Read the model definition and answer for the solid it produces. Units are mm, in the model's axes. A direction names the side the tool comes from. Round coordinates to 2 decimals unless told otherwise and drop trailing zeros. Loops run counter-clockwise (first coordinate to the right, second up) from the corner with the lowest first, then second, coordinate; pieces in that order, holes last. Notation, with made-up numbers: (-16, -38.75) -> (41, -38.75) arc R19 ccw to (41, -31.75) -> close; hole circle Ø7 at (36, -27). An arc over 180 degrees is marked (long way). Put each result on its own line as item: value.
from build123d import *

# Parameters (mm, degrees)
F2_R     = 2.915028
F3_DEPTH = 25.4
F4_SIZE  = 0.8128
F5_R     = 1.809052
F6_DEPTH = 127.001


with BuildPart() as f1:
    # F0 (on Front) → F1 (revolve)
    with BuildSketch(Plane.XZ):
        Polygon((0, -50.8), (0, 0), (0, 76.2), (-6.35, 76.2), (-6.35, 0), (-25.4, 0), align=None)
    revolve(axis=Axis((0, 0, 38.1), (0, 0, -1)))

    # F2 (on face) → F3 (cut)
    with BuildSketch(Plane.XY.offset(76.2)):
        Circle(F2_R)
    extrude(amount=-F3_DEPTH, mode=Mode.SUBTRACT)

    # F4
    f4_edges = [f1.edges().sort_by_distance(p)[0] for p in [
        (6.35, 0, 76.2),
    ]]
    chamfer(f4_edges, length=F4_SIZE)

    # F5 (on face) → F6 (cut, through all)
    with BuildSketch(Plane.XY.offset(76.2)):
        Circle(F5_R)
    extrude(amount=-F6_DEPTH, mode=Mode.SUBTRACT)


solid = f1.part
Item 1: The part is cut by section D-D (z = 7.5). Determine the outline of the cut face in (x, y).
Derived:
outline: circle Ø12.7 at (0, 0); hole circle Ø3.62 at (0, 0)
Item 2: Flat-ended cylindrical pins translate along their axes: pin 1 Ø4 at (x, y) = (16.5, -13) entering from -Z; pin 2 Ø6 at (x, z) = (1.5, 0.5) entering from +Y; pin 3 Ø4 at (x, y) = (19, 14.5) entering from -Z. Find the tip coordinate at first contact, or state that the pin passes through.
Derived:
pin 1: stops at z = -12.79
pin 2: stops at y = 25.4
pin 3: stops at z = -7
Item 3: The part is cut by section A-A (x = 0). Determine the outline of the cut face in (y, z).
Derived:
outline: (-25.4, 0) -> (-1.81, -47.18) -> (-1.81, 50.8) -> (-2.92, 50.8) -> (-2.92, 76.2) -> (-5.54, 76.2) -> (-6.35, 75.39) -> (-6.35, 0) -> close; (1.81, -47.18) -> (25.4, 0) -> (6.35, 0) -> (6.35, 75.39) -> (5.54, 76.2) -> (2.92, 76.2) -> (2.92, 50.8) -> (1.81, 50.8) -> close
Item 4: The part is cut by section C-C (z = -30.5). Determine the outline of the cut face in (x, y).
Derived:
outline: circle Ø20.3 at (0, 0); hole circle Ø3.62 at (0, 0)
Item 5: For a pull along X with two mould halves and no side action, classify faces 1 (the flat face through (5, -5, 0)), 2 (the cylindrical face through (1.38, -6.2, 37.17)), 3 (the flat face through (0, -2, 50.8)) as pulls with the +X half, pulls with the -X half, needs draft (parallel to the pull), parting line crosses it, or undercut.
Derived:
face 1: needs draft
face 2: parting line crosses it
face 3: undercut
Item 6: Which of the six approach directions +Z, -Z, +X, -X, +Y, -Y give full straight-line access (tool end or side, diameter ignored) to faces 4 (the cylindrical face through (-1.436, -1.101, 2.495)), 5 (the cylindrical face through (-0.38, 2.89, 63.68))?
Derived:
face 4: +Z, -Z
face 5: +Z
Item 7: Find the intervals of material crossed by line 1 along X through (y, z) = (0, -23); line 2 along X through (y, z) = (0, -21.5); line 3 along Z through (x, y) = (2, 4), in increasing order.
Derived:
line 1: x = -13.9 to -1.81, 1.81 to 13.9
line 2: x = -14.65 to -1.81, 1.81 to 14.65
line 3: z = -41.86 to 76.2
